The model under review builds one solid part; all positions refer to its coordinate system, in mm. A direction names the side the tool comes from. Give positions to 0.01 mm unless a question says otherwise; leave off trailing zeros. Loops run counter-clockwise (first coordinate to the right, second up) from the corner with the lowest first, then second, coordinate; pieces in that order, holes last. Notation, with made-up numbers: (-11.5, 2.5) - (-1.5, 2.5) arc R15 cw to (-1.5, 15.5) - close; hole circle Ø5 at (56.25, 20). An arc over 180 degrees is marked (long way). Return JSON: item names as keys, results as strings. Group by question number.
```python
from build123d import *

# Parameters (mm, degrees)
SKETCH_0_R         = 7.5
PAD_DEPTH          = 20
POLARPATTERN_COUNT = 3
SKETCH_R           = 10
PAD001_DEPTH       = 15


with BuildPart() as part:
    with BuildSketch(Plane.YZ):
        with BuildLine():
            ThreePointArc((-12.5, 21.650635), (0, -25), (12.5, 21.650635))
            Line((12.5, 91.708438), (12.5, 21.650635))
            ThreePointArc((12.5, 91.708438), (0, 115), (-12.5, 91.708438))
            Line((-12.5, 91.708438), (-12.5, 21.650635))
        make_face()
        Circle(SKETCH_0_R, mode=Mode.SUBTRACT)
    pad = extrude(amount=PAD_DEPTH)

    # PolarPattern: Pad ×3 about axis
    polarpattern_axis = Axis((0, 0, 0), (1, 0, 0))
    for i in range(1, POLARPATTERN_COUNT):
        add(pad.rotate(polarpattern_axis, i * 360 / POLARPATTERN_COUNT))

    with BuildSketch(Plane.YZ):
        with Locations((0, 100)):
            Circle(SKETCH_R)
        with Locations((86.60254, -50)):
            Circle(SKETCH_R)
        with Locations((-86.60254, -50)):
            Circle(SKETCH_R)
    extrude(amount=-PAD001_DEPTH)


solid = part.part
```
1) Draft analysis for pull direction Y (two halves, no side actions). For faces 6 (the face through (-15, 0, 100)), 7 (the face through (-7.395, -1.302, 109.915)), 8 (the face through (-7.395, -81.988, -58.872)), state which applies: +Y half, -Y half, draft (parallel to the pull), parting line (faces both ways), or undercut.
2) We need section C-C, the plane z = 100. Write out the cut boundary in (x, y).
3) We need section B-B, the plane x = 11. Write out the cut boundary in (y, z).
4) We need section D-D, the plane z = -50. Write out the cut boundary in (x, y).
5) For pin 1 Ø5 at (x, z) = (4, -31) entering from -Y; pin 2 Ø16 at (x, z) = (8.5, 44.5) entering from -Y; pin 3 Ø1 at (x, y) = (5, 56.5) entering from +Z, all flat-tipped, find the tip position at first contact; note any pin that passes through.
6) Tool access review of faces 1 (the face through (10, 12.5, 57)), 2 (the face through (-15, 86, -50)), 3 (the face through (-7.4, 95.84, -53.83)), 4 (the face through (10, -12.5, 57)), 5 (the face through (9.86, 43.26, -39.41)): name each direction out of +Z, -Z, +X, -X, +Y, -Y from which nothing blocks a thin tool from reaching the whole face with its end or side.
7) To check wall thickness, follow line 1 (X direction, y = -7, z = 35); line 2 (Y direction, x = 11.5, z = 44.5); line 3 (Z direction, x = 2.5, y = 39). State the ranges of each line that lie inside material, in increasing order.
8) We need section A-A, the plane y = 0. Write out the cut boundary in (x, z), plus the area to 3 significant figures.
Findings:
{
 "1": {"face 6": "draft", "face 7": "parting line", "face 8": "undercut"},
 "2": {"outline": "(-15, -10) - (0, -10) - (0, -15) - (20, -15) - (20, 15) - (0, 15) - (0, 10) - (-15, 10) - close"},
 "3": {"outline": "(-85.67, -35.03) arc R15 ccw (long way) to (-73.17, -56.68) - (-12.5, -21.65) arc R25 ccw to (12.5, -21.65) - (73.17, -56.68) arc R15 ccw (long way) to (85.67, -35.03) - (25, 0) arc R25 ccw to (12.5, 21.65) - (12.5, 91.71) arc R15 ccw (long way) to (-12.5, 91.71) - (-12.5, 21.65) arc R25 ccw to (-25, 0) - close; hole circle Ø15 at (0, 0)"},
 "4": {"outline": "(-15, -96.6) - (0, -96.6) - (0, -101.6) - (20, -101.6) - (20, -61.6) - (0, -61.6) - (0, -76.6) - (-15, -76.6) - close; (-15, 76.6) - (0, 76.6) - (0, 61.6) - (20, 61.6) - (20, 101.6) - (0, 101.6) - (0, 96.6) - (-15, 96.6) - close"},
 "5": {"pin 1": "stops at y = -83.02", "pin 2": "stops at y = -12.5", "pin 3": "stops at z = -17.9"},
 "6": {"face 1": "+X, -X, +Y", "face 2": "+Z, -Z, -X, +Y, -Y", "face 3": "-X", "face 4": "+X, -X, -Y", "face 5": "-Z, +X, -X"},
 "7": {"line 1": "x = 0 to 20", "line 2": "y = -12.5 to 12.5", "line 3": "z = -36.95 to -8.08"},
 "8": {"outline": "(-15, 90) - (0, 90) - (0, 7.5) - (20, 7.5) - (20, 115) - (0, 115) - (0, 110) - (-15, 110) - close; (0, -25) - (20, -25) - (20, -7.5) - (0, -7.5) - close", "area": "2,800 mm^2"}
}
